from build123d import *

# Parameters (mm, degrees)
BOSS_EXTRUDE1_DEPTH = 203.2
CUT_EXTRUDE1_DEPTH  = 316.247758015
CUT_EXTRUDE2_REACH  = 317.248
SKETCH3_W           = 3.556
SKETCH3_H           = 12.7


with BuildPart() as part:
    # Sketch1 → Boss-Extrude1 (new body)
    with BuildSketch(Plane(origin=(0, 0, 0), x_dir=(0, 0, -1), z_dir=(1, 0, 0))):
        Polygon((107.95, -4.33747573), (107.95, -7.524603714), (241.3, 4.142009567), (241.3, 7.329137551), align=None)
    extrude(amount=BOSS_EXTRUDE1_DEPTH)

    # Sketch2 → Cut-Extrude1 (cut, through all)
    with BuildSketch(Plane(origin=(0, -13.677188118, -1.196598909), x_dir=(1, 0, 0), z_dir=(0, 0.9961946980917459, 0.08715574274765497))):
        with BuildLine():
            Line((74.676, 221.335557077), (74.676, 214.985557077))
            ThreePointArc((74.676, 214.985557077), (76.2, 213.461557077), (77.724, 214.985557077))
            Line((77.724, 214.985557077), (77.724, 221.335557077))
            ThreePointArc((77.724, 221.335557077), (76.2, 222.859557077), (74.676, 221.335557077))
        make_face()
        with BuildLine():
            Line((128.524, 221.335557077), (128.524, 214.985557077))
            ThreePointArc((128.524, 214.985557077), (127, 213.461557077), (125.476, 214.985557077))
            Line((125.476, 214.985557077), (125.476, 221.335557077))
            ThreePointArc((125.476, 221.335557077), (127, 222.859557077), (128.524, 221.335557077))
        make_face()
    extrude(amount=-CUT_EXTRUDE1_DEPTH, mode=Mode.SUBTRACT)

    # Sketch3 → Cut-Extrude2 (cut, up to next)
    with BuildSketch(Plane(origin=(0, -13.677188118, -1.196598909), x_dir=(1, 0, 0), z_dir=(0, 0.9961946980917459, 0.08715574274765481)), mode=Mode.PRIVATE) as cut_extrude2_sk1:
        with Locations((8.870592235, 113.286692619)):
            Rectangle(SKETCH3_W, SKETCH3_H)
    cut_extrude2_tool1 = extrude(cut_extrude2_sk1.sketch, amount=-CUT_EXTRUDE2_REACH, mode=Mode.PRIVATE) & part.part
    # Sketch3 → Cut-Extrude2 (cut, up to next)
    with BuildSketch(Plane(origin=(0, -13.677188118, -1.196598909), x_dir=(1, 0, 0), z_dir=(0, 0.9961946980917459, 0.08715574274765481)), mode=Mode.PRIVATE) as cut_extrude2_sk2:
        with Locations((102.088592235, 113.286692619)):
            Rectangle(SKETCH3_W, SKETCH3_H)
    cut_extrude2_tool2 = extrude(cut_extrude2_sk2.sketch, amount=-CUT_EXTRUDE2_REACH, mode=Mode.PRIVATE) & part.part
    # Sketch3 → Cut-Extrude2 (cut, up to next)
    with BuildSketch(Plane(origin=(0, -13.677188118, -1.196598909), x_dir=(1, 0, 0), z_dir=(0, 0.9961946980917459, 0.08715574274765481)), mode=Mode.PRIVATE) as cut_extrude2_sk3:
        with Locations((195.306592235, 113.286692619)):
            Rectangle(SKETCH3_W, SKETCH3_H)
    cut_extrude2_tool3 = extrude(cut_extrude2_sk3.sketch, amount=-CUT_EXTRUDE2_REACH, mode=Mode.PRIVATE) & part.part
    add(cut_extrude2_tool1.solids().sort_by_distance((8.870592, -3.803602, -114.052201))[0], mode=Mode.SUBTRACT)
    add(cut_extrude2_tool2.solids().sort_by_distance((102.088592, -3.803602, -114.052201))[0], mode=Mode.SUBTRACT)
    add(cut_extrude2_tool3.solids().sort_by_distance((195.306592, -3.803602, -114.052201))[0], mode=Mode.SUBTRACT)


solid = part.part
Verification items for the finished model (mm, model axes). A direction names the side the tool comes from. Give positions to 0.01 mm unless a question says otherwise; leave off trailing zeros. Loops run counter-clockwise (first coordinate to the right, second up) from the corner with the lowest first, then second, coordinate; pieces in that order, holes last.
1) Set-up check for faces 1 (the flat face through (0, 0, -174)), 2 (the flat face through (128.524, 4, -219)): record each of +Z, -Z, +X, -X, +Y, -Y from which the full face is reachable in a straight line by a thin tool's end or side.
2) Draft check along Z on faces 3 (the flat face through (100.178, -1.773, -173.692)), 4 (the flat face through (100.178, 1.577, -175.558)), 5 (the flat face through (77.724, 4, -219)). Enter one of: pulls with the +Z half, pulls with the -Z half, needs draft (parallel to the pull), parting line crosses it, or undercut.
3) Sectioned sample at B-B, the plane y = -1. Enter the section's corners in (x, z).
4) Thickness scan on line 1 along X through (y, z) = (-5, -119); line 2 along Y through (x, z) = (25.5, -168); line 3 along Y through (x, z) = (72, -193.5). Record the ranges inside material, lowest first.
5) Depth check by flat-ended pin: pin 1 Ø5 at (x, y) = (153, 2.5) entering from -Z; pin 2 Ø6 at (x, z) = (142, -161) entering from -Y; pin 3 Ø8 at (y, z) = (-4, -224) entering from -X; pin 4 Ø1 at (x, z) = (114, -201.5) entering from +Y. Enter the tip coordinate at first touch or a pass-through.
6) Sectioned sample at A-A, the plane x = 58. Enter the section's corners in (y, z).
Answers:
1. face 1: +Z, -Z, -X, +Y, -Y
1. face 2: +Y, -Y
2. face 3: pulls with the -Z half
2. face 4: pulls with the +Z half
2. face 5: undercut
3. outline: (0, -182.53) - (203.2, -182.53) - (203.2, -146.1) - (0, -146.1) - close
4. line 1: x = 0 to 7.09, 10.65 to 100.31, 103.87 to 193.53, 197.08 to 203.2
4. line 2: y = -2.27 to 0.92
4. line 3: y = -0.04 to 3.15
5. pin 1: stops at z = -241.3
5. pin 2: stops at y = -3.15
5. pin 3: passes through
5. pin 4: stops at y = 3.89
6. outline: (-7.52, -107.95) - (4.14, -241.3) - (7.33, -241.3) - (-4.34, -107.95) - close
